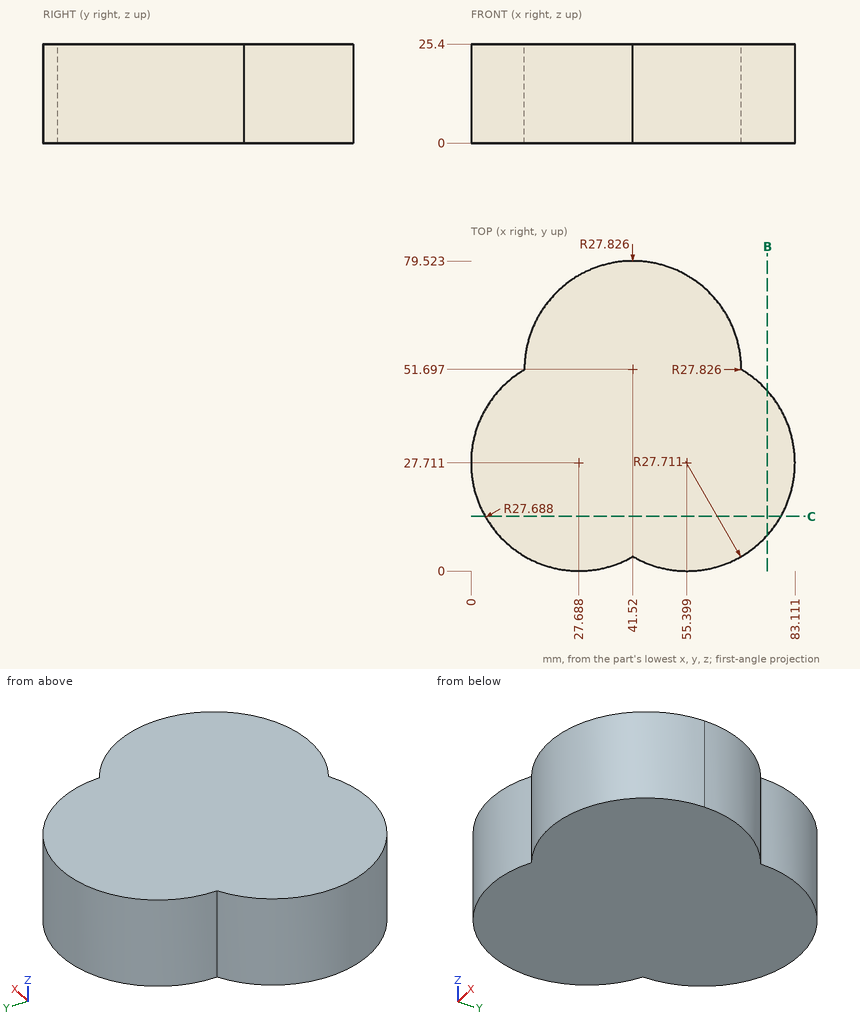
Study the drawing (mm; zero at the part's minimum x, y, z) and answer. Round coordinates to 2 decimals unless told otherwise and drop trailing zeros. Write each loop counter-clockwise with the first axis right and the second up, starting at its lowest first coordinate (ties: lowest second). Pieces come first, ordered by that corner, then holes.
1) Straight lines are drawn through the part: line 1 (Y direction, x = 21, z = 20.5) (1 decimal); line 2 (Y direction, x = 31, z = 18.25); line 3 (X direction, y = 59.5, z = 21.75). For each, find the intervals that lie inside material, in ascending order.
2) Given pin 1 Ø2 at (y, z) = (12, 7) entering from +X; pin 2 Ø4 at (x, z) = (21.5, 21.5) entering from +Y; pin 3 Ø1.5 at (y, z) = (25, 12.5) entering from +X, each flat-ended and moving along its own axis, determine where each tip first touches the part or whether it passes through.
3) A cutting plane is placed at B-B (x = 76). Give the vertices of the cut face in (y, z).
4) A cutting plane is placed at C-C (y = 14). Give the vertices of the cut face in (x, z), plus the area to 3 significant figures.
Completed:
1. line 1: y = 0.8 to 70.5
1. line 2: y = 0.22 to 77.46
1. line 3: x = 14.81 to 68.23
2. pin 1: stops at x = 78.88
2. pin 2: stops at y = 72.9
2. pin 3: stops at x = 83.04
3. outline: (9.18, 0) - (46.25, 0) - (46.25, 25.4) - (9.18, 25.4) - close
4. outline: (3.63, 0) - (79.48, 0) - (79.48, 25.4) - (3.63, 25.4) - close
4. area: 1,930 mm2
